Autodesk Inventor part; units mm, degrees
ref_plane "YZ Plane" through (0, 0, 0) normal (1, 0, 0) x (0, 1, 0)
ref_plane "XZ Plane" through (0, 0, 0) normal (0, 1, 0) x (-1, 0, 0)
ref_plane "XY Plane" through (0, 0, 0) normal (0, 0, 1) x (1, 0, 0)
sketch "Sketch1" plane through (0, 0, 0) normal (0, 0, 1) x (1, 0, 0)
  line L0 (13, -16) -> (-13, -16)
  line L1 (-13, -16) -> (-13, 16)
  line L2 (-13, 16) -> (13, 16)
  line L3 (13, 16) -> (13, -16)
  line L4 (13, -16) -> (-13, 16) construction
  line L5 (-13, -16) -> (13, 16) construction
  circle A0 centre (-9.5, 12) radius 1.6
  circle A1 centre (9.5, -12) radius 1.6
  point P0 (0, 0)
  dimension "d0" = 32
  dimension "d1" = 26
  dimension "d3" = 12
  dimension "d4" = 12
  dimension "d5" = 9.5
  dimension "d6" = 9.5
  dimension "d7" = 3.2
extrude "Extrusion1" add sketch "Sketch1" along normal blind 2
sketch "Sketch2" plane through (0, 0, 2) normal (0, 0, 1) x (1, 0, 0)
  circle A0 centre (0, 0) radius 12
  dimension "d10" = 24
extrude "Extrusion2" add sketch "Sketch2" along normal blind 2.5
fillet "Fillet1" radius 2 4 edges at (-13, 16, 1) (13, 16, 1) (-13, -16, 1) (13, -16, 1)
sketch "Sketch3" plane through (0, 0, 0) normal (0, 0, -1) x (-1, 0, 0)
  line L0 (8, -9.5) -> (-8, -9.5)
  line L1 (-8, -9.5) -> (-8, 9.5)
  line L2 (-8, 9.5) -> (8, 9.5)
  line L3 (8, 9.5) -> (8, -9.5)
  line L4 (8, -9.5) -> (-8, 9.5) construction
  line L5 (-8, -9.5) -> (8, 9.5) construction
  point P0 (0, 0)
  dimension "d14" = 19
  dimension "d15" = 16
extrude "Extrusion3" add sketch "Sketch3" along normal blind 26
sketch "Sketch4" plane through (0, 0, 4.5) normal (0, 0, 1) x (1, 0, 0)
  line L0 (6.5, -2.5) -> (-6.5, -2.5)
  line L1 (-6.5, -2.5) -> (-6.5, 2.5)
  line L2 (-6.5, 2.5) -> (6.5, 2.5)
  line L3 (6.5, 2.5) -> (6.5, -2.5)
  line L4 (6.5, -2.5) -> (-6.5, 2.5) construction
  line L5 (-6.5, -2.5) -> (6.5, 2.5) construction
  point P0 (0, 0)
  dimension "d18" = 13
  dimension "d19" = 5
extrude "Extrusion4" cut sketch "Sketch4" against normal blind 10
properties part number "Delock Panel Connector" material "Aluminum 6061"
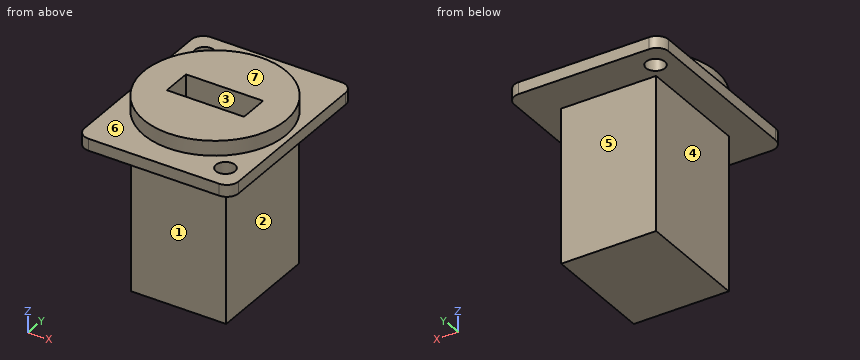
Build history of the part. All positions in model axes, mm. Face numbers are marked on the shaded views. A direction names the side the tool comes from. Coordinates: 2 decimals unless noted, no trailing zeros. Order: outer loops, then holes, each group sorted by start corner. A loop starts at its lowest first (then second) coordinate and runs counter-clockwise, first axis right, second up. Notation, with made-up numbers: (-18, 59.5) - (-10, 59.5) arc R15 ccw to (-10, 68.5) - close; hole circle Ø10 at (15, -21.75). An arc over 180 degrees is marked (long way). Put each result on its own line as item: value.
1. Probe line 1 along Y through (x, z) = (9.5, 0.5); line 2 along X through (y, z) = (-1.5, -3.5); line 3 along Z through (x, y) = (-8.25, 14). List the from-to ranges inside material, lowest first. Write a range as [from, to].
Answer sheet:
line 1: y = [-16, -13.6], [-10.4, 16]
line 2: x = [-8, -6.5], [6.5, 8]
line 3: z = [0, 2]
2. Saw through at D-D (x = 9.5). Write the cut outline in (y, z), and give its area (3 significant figures).
Answer sheet:
outline: (-16, 0) - (-13.6, 0) - (-13.6, 2) - (-16, 2) - close; (-10.4, 0) - (16, 0) - (16, 2) - (7.33, 2) - (7.33, 4.5) - (-7.33, 4.5) - (-7.33, 2) - (-10.4, 2) - close
area: 94.3 mm^2
3. Saw through at C-C (z = -8.5). Write the cut outline in (x, y), and give its area (3 significant figures).
Answer sheet:
outline: (-8, -9.5) - (8, -9.5) - (8, 9.5) - (-8, 9.5) - close
area: 304 mm^2
4. Tool access for the marked faces 4, 5, 6 and 7: list every direction of +Z, -Z, +X, -X, +Y, -Y with a clear straight run to the whole face (end or side of a thin tool).
Answer sheet:
face 4: -Z, -X, +Y, -Y
face 5: -Z, +X, -X, +Y
face 6: +Z
face 7: +Z, +X, -X, +Y, -Y
5. Drop flat-ended pins along their axis: P1, Ø3, axis at x = 9, z = -22.5, coming from the +Y side; P2, Ø3, axis at y = 8.5, z = -9.5, coming from the +X side; P3, Ø5, axis at x = -9.5, y = 12, coming from the -Z side. Give the stop position or say it passes through.
Answer sheet:
P1: stops at y = 9.5
P2: stops at x = 8
P3: stops at z = 0
6. Pull direction Y, two halves, no side cores. Call the marked faces 1, 2 and 3: pulls with the +Y half, pulls with the -Y half, needs draft (parallel to the pull), parting line crosses it, or undercut.
Answer sheet:
face 1: pulls with the -Y half
face 2: needs draft
face 3: undercut
7. Saw through at A-A (x = 0). Write the cut outline in (y, z), and give its area (3 significant figures).
Answer sheet:
outline: (-16, 0) - (-9.5, 0) - (-9.5, -26) - (9.5, -26) - (9.5, 0) - (16, 0) - (16, 2) - (12, 2) - (12, 4.5) - (2.5, 4.5) - (2.5, -5.5) - (-2.5, -5.5) - (-2.5, 4.5) - (-12, 4.5) - (-12, 2) - (-16, 2) - close
area: 568 mm^2
8. Saw through at B-B (y = -12.5). Write the cut outline in (x, z).
Answer sheet:
outline: (-13, 0) - (7.98, 0) - (7.98, 2) - (-13, 2) - close; (11.02, 0) - (13, 0) - (13, 2) - (11.02, 2) - close
